from build123d import *

# Parameters (mm, degrees)
F0_R     = 1.9
F1_DEPTH = 2
F2_DEPTH = 1
F3_R     = 1
F4_DEPTH = 9


with BuildPart() as f1:
    # F0 (on Top) → F1 (new body)
    with BuildSketch(Plane.XY):
        Circle(F0_R)
        Polygon((-0.9006664199, 0), (-0.45033321, 0.78), (0.45033321, 0.78), (0.9006664199, 0), (0.45033321, -0.78), (-0.45033321, -0.78), align=None, mode=Mode.SUBTRACT)
        Polygon((0.45033321, 0.78), (-0.45033321, 0.78), (-0.9006664199, 0), (-0.45033321, -0.78), (0.45033321, -0.78), (0.9006664199, 0), align=None)
    extrude(amount=F1_DEPTH)

    # F0 (on Top) → F2 (cut)
    with BuildSketch(Plane.XY):
        Polygon((0.45033321, 0.78), (-0.45033321, 0.78), (-0.9006664199, 0), (-0.45033321, -0.78), (0.45033321, -0.78), (0.9006664199, 0), align=None)
    extrude(amount=F2_DEPTH, mode=Mode.SUBTRACT)

    # F3 (on face) → F4 (join)
    with BuildSketch(Plane.XY.offset(2)):
        Circle(F3_R)
    extrude(amount=F4_DEPTH)


solid = f1.part
Could you check a few things on this model? Use its own coordinates, in mm. A direction names the side the tool comes from. Give positions to 0.01 mm unless a question says otherwise; leave off trailing zeros. Write each loop counter-clockwise with the first axis right and the second up, starting at its lowest first coordinate (ties: lowest second). Pieces come first, ordered by that corner, then holes. Notation, with made-up numbers: (1.5, 10) - (40.5, 10) arc R9 cw to (40.5, 17) - close; hole circle Ø5 at (64, -18). An arc over 180 degrees is marked (long way). Use CSV: the item, a comma, the result in double quotes. Start each with the question number.
Item 1: If we mould it in two halves opening along X, with no side actions, what happens to faces 1 (the face through (-1.9, 0.08, 0.99)), 2 (the face through (0, 0, 11)), 3 (the face through (0, -0.78, 0.5))? For each: pulls with the +X half, pulls with the -X half, needs draft (parallel to the pull), parting line crosses it, or undercut.
Item 2: I want a section at D-D, the plane x = -1.1. Please give me the cut outline in (y, z), then the cut area to 3 significant figures.
Item 3: I want a section at B-B, the plane y = -0.25. Please give me the cut outline in (x, z), then the cut area to 3 significant figures.
Item 4: For faces 4 (the face through (0, 0.78, 0.5)), 5 (the face through (0, -1, 6)), 6 (the face through (0, -1, 0)), which set-ups out of +Z, -Z, +X, -X, +Y, -Y let a thin tool reach every point of the face, with its end or its side?
Item 5: I want a section at C-C, the plane z = 5.25. Please give me the cut outline in (x, y), then the cut area to 3 significant figures.
Item 6: If I drill on line 1 along Z through (x, y) = (0, -0.7); line 2 along X through (y, z) = (0.1, 1.5); line 3 along Z through (x, y) = (-0.8, 1.5), over which ranges is the centre line in solid material (lowest first)?
Item 7: I want a section at A-A, the plane x = 0. Please give me the cut outline in (y, z), then the cut area to 3 significant figures.
Item 8: I'm going to push a flat-ended pin straight in: pin 1 (2 mm diameter, centred on x = 0.5, z = 7, fed in from -Y). Where does the tip first touch, or does it pass through?
Findings:
1,face 1,"parting line crosses it"
1,face 2,"needs draft"
1,face 3,"undercut"
2,outline,"(-1.55, 0) - (1.55, 0) - (1.55, 2) - (-1.55, 2) - close"
2,area,"6.20 mm2"
3,outline,"(-1.88, 0) - (-0.76, 0) - (-0.76, 1) - (0.76, 1) - (0.76, 0) - (1.88, 0) - (1.88, 2) - (0.97, 2) - (0.97, 11) - (-0.97, 11) - (-0.97, 2) - (-1.88, 2) - close"
3,area,"23.4 mm2"
4,face 4,"-Z"
4,face 5,"+Z"
4,face 6,"-Z, +X, -X, +Y, -Y"
5,outline,"circle Ø2 at (0, 0)"
5,area,"3.14 mm2"
6,line 1,"z = 1 to 11"
6,line 2,"x = -1.9 to 1.9"
6,line 3,"z = 0 to 2"
7,outline,"(-1.9, 0) - (-0.78, 0) - (-0.78, 1) - (0.78, 1) - (0.78, 0) - (1.9, 0) - (1.9, 2) - (1, 2) - (1, 11) - (-1, 11) - (-1, 2) - (-1.9, 2) - close"
7,area,"24.0 mm2"
8,pin 1,"stops at y = -1"
